Design review of the part built by this model. Coordinates are the model's own, in mm. Face numbers are marked on the shaded views. A direction names the side the tool comes from. Give positions to 0.01 mm unless a question says otherwise; leave off trailing zeros. Order: outer loops, then holes, each group sorted by start corner. A loop starts at its lowest first (then second) coordinate and runs counter-clockwise, first axis right, second up. Notation, with made-up numbers: M 46.25,72 L 72.25,72 A24 ccw 72.25,106 Z; hole C -37.75,-2.75 d6. An arc over 180 degrees is marked long. Answer as a JSON object with one key per item and string values.
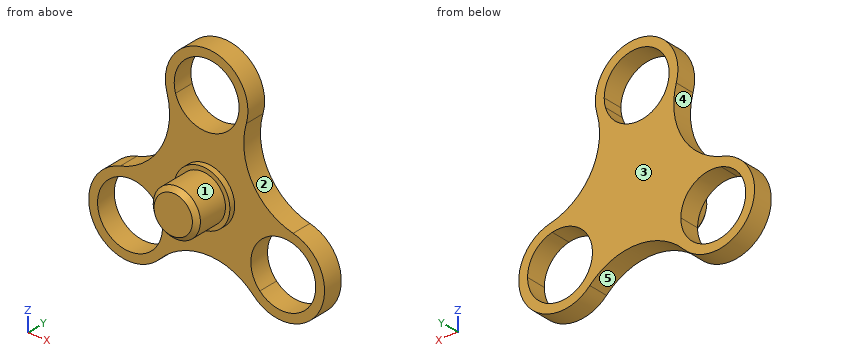
from build123d import *

# Parameters (mm, degrees)
F0_R     = 11
F1_DEPTH = 7
F2_SCALE = 0.5
F5_R     = 4.75
F5_R_2   = 4
F6_DEPTH = 1
F7_SIZE  = 0.75


with BuildPart() as f1:
    # F0 (on Front) → F1 (new body)
    with BuildSketch(Plane.XZ):
        with BuildLine():
            ThreePointArc((29.3216524239, -1.4044694133), (15.5190640284, 8.9599357944), (13.4445200212, 26.0955305867))
            ThreePointArc((13.4445200212, 26.0955305867), (0, 44), (-13.4445200212, 26.0955305867))
            ThreePointArc((-13.4445200212, 26.0955305867), (-15.5190640284, 8.9599357944), (-29.3216524239, -1.4044694133))
            ThreePointArc((-29.3216524239, -1.4044694133), (-38.1051177665, -22), (-15.8771324027, -24.6910611734))
            ThreePointArc((-15.8771324027, -24.6910611734), (0, -17.9198715888), (15.8771324027, -24.6910611734))
            ThreePointArc((15.8771324027, -24.6910611734), (38.1051177665, -22), (29.3216524239, -1.4044694133))
        make_face()
        with BuildLine():
            ThreePointArc((11, 30), (10.8903412687, 28.4506559287), (10.5635514452, 26.9322026038))
            ThreePointArc((10.5635514452, 26.9322026038), (12.9209878171, 7.4599357944), (28.6057473574, -4.3177973962))
            ThreePointArc((28.6057473574, -4.3177973962), (34.6374022725, -8.2130580407), (36.9807621135, -15))
            ThreePointArc((36.9807621135, -15), (30.084161423, -25.2059842302), (18.0421959122, -22.6144052077))
            ThreePointArc((18.0421959122, -22.6144052077), (0, -14.9198715888), (-18.0421959122, -22.6144052077))
            ThreePointArc((-18.0421959122, -22.6144052077), (-35.5070415552, -20.5), (-28.6057473574, -4.3177973962))
            ThreePointArc((-28.6057473574, -4.3177973962), (-12.9209878171, 7.4599357944), (-10.5635514452, 26.9322026038))
            ThreePointArc((-10.5635514452, 26.9322026038), (-1.5493440713, 40.8903412687), (11, 30))
        make_face(mode=Mode.SUBTRACT)
        with BuildLine():
            ThreePointArc((28.6057473574, -4.3177973962), (12.9209878171, 7.4599357944), (10.5635514452, 26.9322026038))
            ThreePointArc((10.5635514452, 26.9322026038), (0, 19), (-10.5635514452, 26.9322026038))
            ThreePointArc((-10.5635514452, 26.9322026038), (-12.9209878171, 7.4599357944), (-28.6057473574, -4.3177973962))
            ThreePointArc((-28.6057473574, -4.3177973962), (-19.1938201542, -6.3433598411), (-14.9807621135, -15))
            ThreePointArc((-14.9807621135, -15), (-15.7747778833, -19.1033993094), (-18.0421959122, -22.6144052077))
            ThreePointArc((-18.0421959122, -22.6144052077), (0, -14.9198715888), (18.0421959122, -22.6144052077))
            ThreePointArc((18.0421959122, -22.6144052077), (16.4544826719, -9.5), (28.6057473574, -4.3177973962))
        make_face()
        Circle(F0_R, mode=Mode.SUBTRACT)
    extrude(amount=F1_DEPTH)


with BuildPart() as f1_1:
    # F2: moved
    add(f1.part.scale(F2_SCALE))

    # F3 (on Right) → F4 (revolve)
    with BuildSketch(Plane.YZ):
        Polygon((-10.5, -4), (-3.5, -4), (-3.5, -0.7022347066), (-3.5, 0), (-10.5, 0), align=None)
        Polygon((-3.5, -4), (-3.5, -5.5), (0, -5.5), (0, 0), (-3.5, 0), (-3.5, -0.7022347066), align=None)
    revolve(axis=Axis((0, -7, 0), (0, -1, 0)))

    # F5 (on face) → F6 (join)
    with BuildSketch(Plane.XZ.offset(3.5)):
        Circle(F5_R)
        Circle(F5_R_2, mode=Mode.SUBTRACT)
    extrude(amount=F6_DEPTH)

    # F7
    f7_edges = [f1_1.edges().sort_by_distance(p)[0] for p in [
        (0, -10.5, 4),
    ]]
    chamfer(f7_edges, length=F7_SIZE)


solid = f1_1.part
(1) To check wall thickness, follow L1, parallel to X at y = -1.4, z = -7.5; L2, parallel to X at y = -1.1, z = 15; L3, parallel to Z at x = -16, y = -2.75. State the ranges of each line that lie inside material, in increasing order. Write a range as from..to.
Checked values:
{"L1": "x = -19.99..-18.49, -7.49..7.49, 18.49..19.99", "L2": "x = -7..-5.5, 5.5..7", "L3": "z = -13.82..-12.1, -2.9..-1.18"}
(2) We need section C-C (z = 0). Write out the cut boundary in (x, y), plus the area to 3 significant figures.
Checked values:
{"outline": "M -12.66,-3.5 L -4.75,-3.5 L -4.75,-4.5 L -4,-4.5 L -4,-9.75 L -3.25,-10.5 L 3.25,-10.5 L 4,-9.75 L 4,-4.5 L 4.75,-4.5 L 4.75,-3.5 L 12.66,-3.5 L 12.66,0 L -12.66,0 Z", "area": "146 mm^2"}
(3) Tool access review of the marked faces 1 and 2: name each direction out of +Z, -Z, +X, -X, +Y, -Y from which nothing blocks a thin tool from reaching the whole face with its end or side.
Checked values:
{"face 1": "-Y", "face 2": "+X, +Y, -Y"}
(4) Draft analysis for pull direction X (two halves, no side actions). For the marked faces 3, 4 and 5, state which applies: +X half, -X half, draft (parallel to the pull), parting line (faces both ways), or undercut.
Checked values:
{"face 3": "draft", "face 4": "-X half", "face 5": "undercut"}
(5) Insertion check: pin 1 (3 mm diameter, centred on y = -6.5, z = 10.5, fed in from -X); pin 2 (1.5 mm diameter, centred on y = -7, z = -1.5, fed in from -X); pin 3 (6 mm diameter, centred on x = -7.5, y = -1.5, fed in from -Z); pin 4 (14.5 mm diameter, centred on x = -12.99, z = -7.5, fed in from -Y). Each pin has a flat end and moves straight along its axis. Give the tip position at first contact, or say it passes through.
Checked values:
{"pin 1": "passes through", "pin 2": "stops at x = -3.93", "pin 3": "stops at z = -14.04", "pin 4": "stops at y = -3.5"}
(6) We need section A-A (x = 0). Write out the cut boundary in (y, z), plus the area to 3 significant figures.
Checked values:
{"outline": "M -10.5,-3.25 L -9.75,-4 L -4.5,-4 L -4.5,-4.75 L -3.5,-4.75 L -3.5,-8.96 L 0,-8.96 L 0,9.5 L -3.5,9.5 L -3.5,4.75 L -4.5,4.75 L -4.5,4 L -9.75,4 L -10.5,3.25 Z; M -3.5,20.5 L 0,20.5 L 0,22 L -3.5,22 Z", "area": "127 mm^2"}
(7) We need section D-D (x = 17). Write out the cut boundary in (y, z), plus the area to 3 significant figures.
Checked values:
{"outline": "M -3.5,-13.24 L 0,-13.24 L 0,-11.26 L -3.5,-11.26 Z; M -3.5,-3.74 L 0,-3.74 L 0,-1.76 L -3.5,-1.76 Z", "area": "13.8 mm^2"}
(8) We need section B-B (z = 17.5). Write out the cut boundary in (x, y).
Checked values:
{"outline": "M -6.54,-3.5 L -4.9,-3.5 L -4.9,0 L -6.54,0 Z; M 4.9,-3.5 L 6.54,-3.5 L 6.54,0 L 4.9,0 Z"}
